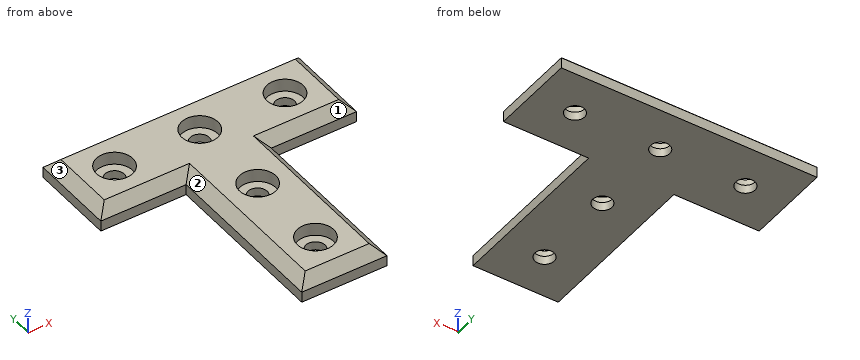
from build123d import *

# Parameters (mm, degrees)
F0_R     = 2.25
F1_DEPTH = 5
F2_SIZE  = 2.5
F3_R     = 4.25
F3_R_2   = 2.25
F4_DEPTH = 3


with BuildPart() as f1:
    # F0 (on Top) → F1 (new body)
    with BuildSketch(Plane.XY):
        Polygon((-10, -50), (0, -50), (10, -50), (10, -10), (30, -10), (30, 10), (0, 10), (-30, 10), (-30, -10), (-10, -10), align=None)
        with Locations((0, -40)):
            Circle(F0_R, mode=Mode.SUBTRACT)
        with Locations((-20, 0)):
            Circle(F0_R, mode=Mode.SUBTRACT)
        with Locations((0, -20)):
            Circle(F0_R, mode=Mode.SUBTRACT)
        Circle(F0_R, mode=Mode.SUBTRACT)
        with Locations((20, 0)):
            Circle(F0_R, mode=Mode.SUBTRACT)
    extrude(amount=F1_DEPTH)

    # F2
    f2_edges = [f1.edges().sort_by_distance(p)[0] for p in [
        (0, -50, 5),
        (10, -30, 5),
        (20, -10, 5),
        (30, 0, 5),
        (0, 10, 5),
        (-30, 0, 5),
        (-20, -10, 5),
        (-10, -30, 5),
    ]]
    chamfer(f2_edges, length=F2_SIZE)

    # F3 (on face) → F4 (cut)
    with BuildSketch(Plane.XY.offset(5)):
        with Locations((-20, 0)):
            Circle(F3_R)
        with Locations((-20, 0)):
            Circle(F3_R_2, mode=Mode.SUBTRACT)
        Circle(F3_R)
        Circle(F3_R_2, mode=Mode.SUBTRACT)
        with Locations((20, 0)):
            Circle(F3_R)
        with Locations((20, 0)):
            Circle(F3_R_2, mode=Mode.SUBTRACT)
        with Locations((0, -20)):
            Circle(F3_R)
        with Locations((0, -20)):
            Circle(F3_R_2, mode=Mode.SUBTRACT)
        with Locations((0, -40)):
            Circle(F3_R)
        with Locations((0, -40)):
            Circle(F3_R_2, mode=Mode.SUBTRACT)
    extrude(amount=-F4_DEPTH, mode=Mode.SUBTRACT)


solid = f1.part
Geometry: final body of the model. Coordinates: model frame, mm. Face numbers are marked on the shaded views. A direction names the side the tool comes from. Coordinates: 2 decimals unless noted, no trailing zeros. Loops run counter-clockwise (first coordinate to the right, second up) from the corner with the lowest first, then second, coordinate; pieces in that order, holes last. Notation, with made-up numbers: M 10,67.5 L 39,67.5 A7 cw 39,79.5 Z; hole C -20.5,27 d8. An arc over 180 degrees is marked long. One line per item, written item: value. Start each with the question number.
1) Cut plane C-C (y = 0). Count the separate pieces of the cut face and the enclosed holes in it, then the cut area to 3 significant figures.
2) Cut plane A-A (x = -20). Return loops of the section in (y, z), then the cut area to 4 significant figures.
3) Cut plane D-D (z = 3.65). Return loops of the section in (x, y), then the cut area to 3 significant figures.
4) Reachability of the marked faces 1, 2 and 3 from +Z, -Z, +X, -X, +Y, -Y: full face, straight path, thin tool, end or side. Return the list, or none.
5) Material intervals for L1, parallel to Y at x = 0, z = 0.65; L2, parallel to Y at x = 0, z = 3.9; L3, parallel to Y at x = 20, z = 0.4, sorted ascending. Write a range as from..to.
6) Pin query (flat end, axial travel): P1, Ø0.8, axis at x = -22.5, z = 1, coming from the -Y side; P2, Ø7.5, axis at x = 0, y = 0, coming from the +Z side. Return the tip coordinate at first contact, or that it passes through.
Evaluation:
1. separate pieces: 4
1. enclosed holes: 0
1. area: 190 mm^2
2. outline: M -10,0 L -2.25,0 L -2.25,2 L -4.25,2 L -4.25,5 L -7.5,5 L -10,2.5 Z; M 2.25,0 L 10,0 L 10,2.5 L 7.5,5 L 4.25,5 L 4.25,2 L 2.25,2 Z
2. area: 59.25 mm^2
3. outline: M -28.85,-8.85 L -8.85,-8.85 L -8.85,-48.85 L 8.85,-48.85 L 8.85,-8.85 L 28.85,-8.85 L 28.85,8.85 L -28.85,8.85 Z; hole C -20,0 d8.5; hole C 0,-40 d8.5; hole C 0,-20 d8.5; hole C 0,0 d8.5; hole C 20,0 d8.5
3. area: 1,450 mm^2
4. face 1: +Z, +X, -Y
4. face 2: +Z, -X, -Y
4. face 3: +Z, -X, +Y, -Y
5. L1: -50..-42.25, -37.75..-22.25, -17.75..-2.25, 2.25..10
5. L2: -48.6..-44.25, -35.75..-24.25, -15.75..-4.25, 4.25..8.6
5. L3: -10..-2.25, 2.25..10
6. P1: y = -10
6. P2: z = 2
